Design review of the part shown in the three views and the two pictorial views. Dimensions are in mm from the part's minimum x, y and z. A direction names the side the tool comes from. Round coordinates to 2 decimals unless told otherwise and drop trailing zeros. Loops run counter-clockwise (first coordinate to the right, second up) from the corner with the lowest first, then second, coordinate; pieces in that order, holes last.
1. Consider section B-B on z = 8. State the section outline as (x, y) points.
2. Draft analysis for pull direction Y (two halves, no side actions). For the marked faces 1, 2, 3 and 4, state which applies: released by +Y, released by -Y, zero draft, split by the parting line, or undercut.
3. To check wall thickness, follow line 1 along Y through (x, z) = (7.75, 9.5); line 2 along X through (y, z) = (3.5, 16.5) (1 decimal); line 3 along Y through (x, z) = (3.75, 20.75) (1 decimal). State the ranges of each line that lie inside material, in increasing order.
4. Consider section D-D on z = 23.75. State the section outline as (x, y) points.
5. Consider section C-C on y = 14.5. State the section outline as (x, z) points.
6. Tool access review of the marked faces 5 and 6: name each direction out of +Z, -Z, +X, -X, +Y, -Y from which nothing blocks a thin tool from reaching the whole face with its end or side.
7. Consider section A-A on x = 8.25. State the section outline as (y, z) points.
8. Clearance check with flat-ended pins moving along their axes: pin 1 Ø1.3 at (x, y) = (5, 16.84) entering from +Z; pin 2 Ø1.5 at (x, y) = (14, 10.5) entering from -Z. State where each tip first meets the part, or that it passes through.
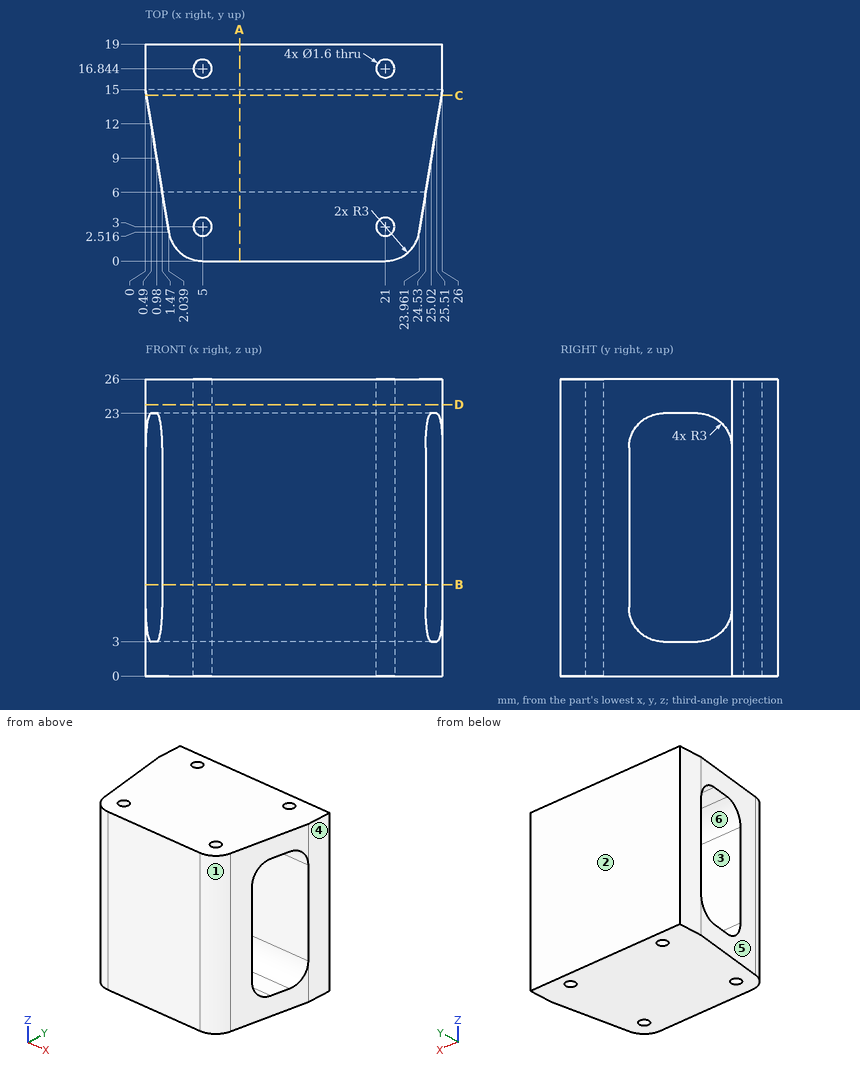
Resolved:
1. outline: (0, 15) - (26, 15) - (26, 19) - (0, 19) - close; (1.47, 6) - (2.04, 2.52) arc R3 ccw to (5, 0) - (21, 0) arc R3 ccw to (23.96, 2.52) - (24.53, 6) - close; hole circle Ø1.6 at (5, 3); hole circle Ø1.6 at (5, 16.84); hole circle Ø1.6 at (21, 3); hole circle Ø1.6 at (21, 16.84)
2. face 1: released by -Y
2. face 2: released by +Y
2. face 3: undercut
2. face 4: zero draft
3. line 1: y = 0 to 6, 15 to 19
3. line 2: x = 1.9 to 4.4, 5.6 to 20.4, 21.6 to 24.1
3. line 3: y = 0.3 to 6.1, 14.9 to 19
4. outline: (0, 15) - (2.04, 2.52) arc R3 ccw to (5, 0) - (21, 0) arc R3 ccw to (23.96, 2.52) - (26, 15) - (26, 19) - (0, 19) - close; hole circle Ø1.6 at (5, 3); hole circle Ø1.6 at (5, 16.84); hole circle Ø1.6 at (21, 3); hole circle Ø1.6 at (21, 16.84)
5. outline: (0.08, 0) - (25.92, 0) - (25.92, 4.34) - (0.08, 4.34) - close; (0.08, 21.66) - (25.92, 21.66) - (25.92, 26) - (0.08, 26) - close
6. face 5: +Z, -Z, -X, -Y
6. face 6: +X, -X
7. outline: (0, 0) - (19, 0) - (19, 26) - (0, 26) - close; hole (6, 6) arc R3 ccw to (9, 3) - (12, 3) arc R3 ccw to (15, 6) - (15, 20) arc R3 ccw to (12, 23) - (9, 23) arc R3 ccw to (6, 20) - close
8. pin 1: passes through
8. pin 2: stops at z = 0
